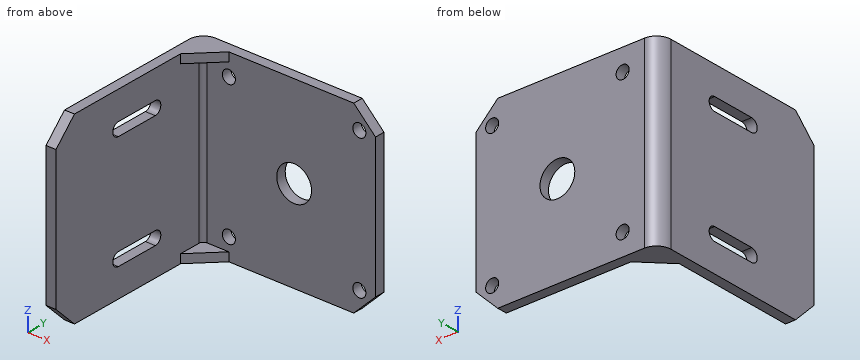
from build123d import *

# Parameters (mm, degrees)
BRIDA_BASE1_DEPTH       = 42
CHAFL_N1_SIZE           = 5
CORTAR_EXTRUIR1_REACH   = 74.746
CROQUIS6_R              = 1.5
CROQUIS6_R_2            = 4
CORTAR_EXTRUIR2_REACH   = 73.448
SALIENTE_EXTRUIR1_START = -2
SALIENTE_EXTRUIR1_DEPTH = 2


# Sheet-metal steps are written as plain solids
with BuildPart() as part:
    # Croquis1 → Brida base1 (new body)
    with BuildSketch(Plane.XY):
        with BuildLine():
            Line((0, 0), (0, 38.71))
            ThreePointArc((0, 38.71), (0.96361869, 41.03638131), (3.29, 42))
            Line((3.29, 42), (42, 42))
            Line((42, 42), (42, 39.71))
            Line((42, 39.71), (3.29, 39.71))
            ThreePointArc((3.29, 39.71), (2.582893219, 39.417106781), (2.29, 38.71))
            Line((2.29, 38.71), (2.29, 0))
            Line((2.29, 0), (0, 0))
        make_face()
    extrude(amount=BRIDA_BASE1_DEPTH)

    # Chaflán1
    chafl_n1_edges = [part.edges().sort_by_distance(p)[0] for p in [
        (1.145, 0, 42),
        (1.145, 0, 0),
        (42, 40.855, 42),
        (42, 40.855, 0),
    ]]
    chamfer(chafl_n1_edges, length=CHAFL_N1_SIZE)

    # Croquis6 → Cortar-Extruir1 (cut, up to next)
    with BuildSketch(Plane(origin=(0, 42, 0), x_dir=(1, 0, 0), z_dir=(0, 1, 0)), mode=Mode.PRIVATE) as cortar_extruir1_sk1:
        with Locations(Location((8.29, -5, 0), (0, 0, 270))):
            Circle(CROQUIS6_R)
    cortar_extruir1_tool1 = extrude(cortar_extruir1_sk1.sketch, amount=-CORTAR_EXTRUIR1_REACH, mode=Mode.PRIVATE) & part.part
    # Croquis6 → Cortar-Extruir1 (cut, up to next)
    with BuildSketch(Plane(origin=(0, 42, 0), x_dir=(1, 0, 0), z_dir=(0, 1, 0)), mode=Mode.PRIVATE) as cortar_extruir1_sk2:
        with Locations(Location((38.29, -5, 0), (0, 0, 270))):
            Circle(CROQUIS6_R)
    cortar_extruir1_tool2 = extrude(cortar_extruir1_sk2.sketch, amount=-CORTAR_EXTRUIR1_REACH, mode=Mode.PRIVATE) & part.part
    # Croquis6 → Cortar-Extruir1 (cut, up to next)
    with BuildSketch(Plane(origin=(0, 42, 0), x_dir=(1, 0, 0), z_dir=(0, 1, 0)), mode=Mode.PRIVATE) as cortar_extruir1_sk3:
        with Locations(Location((38.29, -37, 0), (0, 0, 270))):
            Circle(CROQUIS6_R)
    cortar_extruir1_tool3 = extrude(cortar_extruir1_sk3.sketch, amount=-CORTAR_EXTRUIR1_REACH, mode=Mode.PRIVATE) & part.part
    # Croquis6 → Cortar-Extruir1 (cut, up to next)
    with BuildSketch(Plane(origin=(0, 42, 0), x_dir=(1, 0, 0), z_dir=(0, 1, 0)), mode=Mode.PRIVATE) as cortar_extruir1_sk4:
        with Locations(Location((8.29, -37, 0), (0, 0, 270))):
            Circle(CROQUIS6_R)
    cortar_extruir1_tool4 = extrude(cortar_extruir1_sk4.sketch, amount=-CORTAR_EXTRUIR1_REACH, mode=Mode.PRIVATE) & part.part
    # Croquis6 → Cortar-Extruir1 (cut, up to next)
    with BuildSketch(Plane(origin=(0, 42, 0), x_dir=(1, 0, 0), z_dir=(0, 1, 0)), mode=Mode.PRIVATE) as cortar_extruir1_sk5:
        with Locations(Location((23.29, -21, 0), (0, 0, 270))):
            Circle(CROQUIS6_R_2)
    cortar_extruir1_tool5 = extrude(cortar_extruir1_sk5.sketch, amount=-CORTAR_EXTRUIR1_REACH, mode=Mode.PRIVATE) & part.part
    add(cortar_extruir1_tool1.solids().sort_by_distance((8.29, 42, 5))[0], mode=Mode.SUBTRACT)
    add(cortar_extruir1_tool2.solids().sort_by_distance((38.29, 42, 5))[0], mode=Mode.SUBTRACT)
    add(cortar_extruir1_tool3.solids().sort_by_distance((38.29, 42, 37))[0], mode=Mode.SUBTRACT)
    add(cortar_extruir1_tool4.solids().sort_by_distance((8.29, 42, 37))[0], mode=Mode.SUBTRACT)
    add(cortar_extruir1_tool5.solids().sort_by_distance((23.29, 42, 21))[0], mode=Mode.SUBTRACT)

    # Croquis7 → Cortar-Extruir2 (cut, up to next)
    with BuildSketch(Plane(origin=(2.29, 0, 0), x_dir=(0, 0, -1), z_dir=(1, 0, 0)), mode=Mode.PRIVATE) as cortar_extruir2_sk1:
        with BuildLine():
            Line((-35.5, 16.855), (-35.5, 26.855))
            ThreePointArc((-35.5, 26.855), (-34, 28.355), (-32.5, 26.855))
            Line((-32.5, 26.855), (-32.5, 16.855))
            ThreePointArc((-32.5, 16.855), (-34, 15.355), (-35.5, 16.855))
        make_face()
    cortar_extruir2_tool1 = extrude(cortar_extruir2_sk1.sketch, amount=-CORTAR_EXTRUIR2_REACH, mode=Mode.PRIVATE) & part.part
    # Croquis7 → Cortar-Extruir2 (cut, up to next)
    with BuildSketch(Plane(origin=(2.29, 0, 0), x_dir=(0, 0, -1), z_dir=(1, 0, 0)), mode=Mode.PRIVATE) as cortar_extruir2_sk2:
        with BuildLine():
            Line((-6.5, 16.855), (-6.5, 26.855))
            ThreePointArc((-6.5, 26.855), (-8, 28.355), (-9.5, 26.855))
            Line((-9.5, 26.855), (-9.5, 16.855))
            ThreePointArc((-9.5, 16.855), (-8, 15.355), (-6.5, 16.855))
        make_face()
    cortar_extruir2_tool2 = extrude(cortar_extruir2_sk2.sketch, amount=-CORTAR_EXTRUIR2_REACH, mode=Mode.PRIVATE) & part.part
    add(cortar_extruir2_tool1.solids().sort_by_distance((2.29, 21.855, 34))[0], mode=Mode.SUBTRACT)
    add(cortar_extruir2_tool2.solids().sort_by_distance((2.29, 21.855, 8))[0], mode=Mode.SUBTRACT)

    # Croquis9 → Saliente-Extruir1 (add)
    with BuildSketch(Plane.XY.offset(42).offset(SALIENTE_EXTRUIR1_START)):
        with BuildLine():
            Line((2.29, 38.71), (2.29, 33.71))
            Line((2.29, 33.71), (8.29, 39.71))
            Line((8.29, 39.71), (3.29, 39.71))
            ThreePointArc((3.29, 39.71), (2.582893219, 39.417106781), (2.29, 38.71))
        make_face()
    saliente_extruir1 = extrude(amount=SALIENTE_EXTRUIR1_DEPTH)

    # Simetría1: Saliente-Extruir1 across plane
    add(saliente_extruir1.mirror(Plane.XY.offset(21)))


solid = part.part
For this review, take the finished solid that the model builds, in its own axes (mm). Round coordinates to 2 decimals unless told otherwise and drop trailing zeros. Order: outer loops, then holes, each group sorted by start corner. A loop starts at its lowest first (then second) coordinate and runs counter-clockwise, first axis right, second up. Notation, with made-up numbers: M 55.5,-11.75 L 104.5,-11.75 A27 ccw 104.5,14.25 Z; hole C 53.5,-20.75 d3. An arc over 180 degrees is marked long. Use a Markdown table: item, result. Add a question column.
Item 1: To check wall thickness, follow line 1 along Z through (x, y) = (38, 40); line 2 along X through (y, z) = (40.4, 37); line 3 along X through (y, z) = (11.5, 37). State the ranges of each line that lie inside material, in increasing order.
Item 2: Add section D-D, the plane x = 38.29. Give the boundary of the cut face in (y, z), then the cut area to 3 significant figures.
Item 3: Insertion check: pin 1 (12 mm diameter, centred on x = 32, z = 20, fed in from -Y); pin 2 (4 mm diameter, centred on x = 38.29, z = 5, fed in from +Y); pin 3 (11.5 mm diameter, centred on y = 28, z = 28, fed in from +X). Each pin has a flat end and moves straight along its axis. Give the tip position at first contact, or say it passes through.
Item 4: Add section B-B, the plane z = 34. Give the boundary of the cut face in (x, y) (3 decimals), then the cut area to 3 significant figures.
Item 5: Add section A-A, the plane y = 25.5. Give the boundary of the cut face in (x, z).
Item 6: Add section C-C, the plane x = 23.29. Give the boundary of the cut face in (y, z).
Geometry results:
| question | item | result |
|---|---|---|
| 1 | line 1 | z = 1 to 3.53, 6.47 to 35.53, 38.47 to 41 |
| 1 | line 2 | x = 0.47 to 6.79, 9.79 to 36.79, 39.79 to 42 |
| 1 | line 3 | x = 0 to 2.29 |
| 2 | outline | M 39.71,1.29 L 42,1.29 L 42,3.5 L 39.71,3.5 Z; M 39.71,6.5 L 42,6.5 L 42,35.5 L 39.71,35.5 Z; M 39.71,38.5 L 42,38.5 L 42,40.71 L 39.71,40.71 Z |
| 2 | area | 76.5 mm² |
| 3 | pin 1 | stops at y = 39.71 |
| 3 | pin 2 | stops at y = 42 |
| 3 | pin 3 | stops at x = 2.29 |
| 4 | outline | M 0,0 L 2.29,0 L 2.29,15.355 L 0,15.355 Z; M 0,28.355 L 2.29,28.355 L 2.29,38.71 A1 cw 3.29,39.71 L 42,39.71 L 42,42 L 3.29,42 A3.29 ccw 0,38.71 Z |
| 4 | area | 155 mm² |
| 5 | outline | M 0,0 L 2.29,0 L 2.29,6.5 L 0,6.5 Z; M 0,9.5 L 2.29,9.5 L 2.29,32.5 L 0,32.5 Z; M 0,35.5 L 2.29,35.5 L 2.29,42 L 0,42 Z |
| 6 | outline | M 39.71,0 L 42,0 L 42,17 L 39.71,17 Z; M 39.71,25 L 42,25 L 42,42 L 39.71,42 Z |
